Model file for the job. Use its own axes, mm. A direction names the side the tool comes from. Round coordinates to 2 decimals unless told otherwise and drop trailing zeros. Order: outer loops, then holes, each group sorted by start corner. A loop starts at its lowest first (then second) coordinate and runs counter-clockwise, first axis right, second up. Notation, with made-up numbers: (25, -7.75) - (36, -7.75) arc R17 ccw to (36, 12.25) - close; hole circle Ø9 at (-28.75, 44.25). An arc over 180 degrees is marked (long way). Put each result on its own line as item: value. Start each with the question number.
Item 1: Saw through at C-C on x = 100. List the corners of the cut face in (y, z).
Item 2: Which spindle directions (+Z, -Z, +X, -X, +Y, -Y) get a long thin tool onto all of the face, cutting with end or side? Do faces 1 (the face through (80, 14, 0)), 2 (the face through (80, 12.5, -82)). Say none if no direction does.
Item 3: Probe probe 1 along Z at (x, y) = (130, 8.5); probe 2 along X at (y, z) = (8.75, -9); probe 3 along Z at (x, y) = (19.5, 17.5). List the from-to ranges inside material, lowest first.
Item 4: Pin check, flat tip, straight feed: pin 1 Ø12 at (x, z) = (85.5, -82.5) entering from +Y. Stop position of the tip, or through.
Item 5: Saw through at A-A on z = -43. List the corners of the cut face in (x, y).
Item 6: Saw through at B-B on y = 19.75. List the corners of the cut face in (x, z), plus the area to 4 significant figures.
Item 7: Mould opens along X. For faces 3 (the face through (0, 14, -82)), 4 (the face through (80, 10, -11.5)), 5 (the face through (82, 1, -2)) say: pulls with the +X half, pulls with the -X half, needs draft (parallel to the pull), parting line crosses it, or undercut.
```python
from build123d import *

# Parameters (mm, degrees)
SKETCH1_W           = 162
SKETCH1_H           = 162
SKETCH1_W_2         = 140
SKETCH1_H_2         = 140
BOSS_EXTRUDE1_DEPTH = 7.5
SKETCH2_W           = 139
SKETCH2_H           = 139
BOSS_EXTRUDE2_DEPTH = 5
FILLET1_R           = 5
BOSS_EXTRUDE3_START = 15
BOSS_EXTRUDE3_DEPTH = 15


with BuildPart() as part:
    # Sketch1 → Boss-Extrude1 (new body)
    # profile 1 of 2: a face of its own
    with BuildSketch(Plane(origin=(0, 0, 0), x_dir=(1, 0, 0), z_dir=(0, 1, 0))):
        with Locations((81, 81)):
            Rectangle(SKETCH1_W, SKETCH1_H)
        with Locations((81, 81)):
            Rectangle(SKETCH1_W_2, SKETCH1_H_2, mode=Mode.SUBTRACT)
    # profile 2 of 2: a face of its own
    with BuildSketch(Plane(origin=(0, 0, 0), x_dir=(1, 0, 0), z_dir=(0, 1, 0))):
        with Locations((81, 81)):
            Rectangle(SKETCH1_W_2, SKETCH1_H_2)
    extrude(amount=BOSS_EXTRUDE1_DEPTH)

    # Sketch2 → Boss-Extrude2 (add)
    with BuildSketch(Plane(origin=(0, 7.5, 0), x_dir=(1, 0, 0), z_dir=(0, 1, 0))):
        with Locations((81, 81)):
            Rectangle(SKETCH2_W, SKETCH2_H)
    extrude(amount=BOSS_EXTRUDE2_DEPTH)

    # Fillet1
    fillet1_edges = [part.edges().sort_by_distance(p)[0] for p in [
        (11.5, 10, -150.5),
        (11.5, 10, -11.5),
        (150.5, 10, -11.5),
        (150.5, 10, -150.5),
        (0, 0, -81),
        (81, 0, -162),
        (162, 0, -81),
        (81, 0, 0),
        (0, 3.75, 0),
        (0, 3.75, -162),
        (162, 3.75, -162),
        (162, 3.75, 0),
    ]]
    fillet(fillet1_edges, radius=FILLET1_R)

    # Sketch3 → Boss-Extrude3 (add)
    with BuildSketch(Plane(origin=(0, 7.5, 0), x_dir=(1, 0, 0), z_dir=(0, 1, 0)).offset(BOSS_EXTRUDE3_START)):
        with BuildLine():
            ThreePointArc((5, 162), (1.464466094, 160.535533906), (0, 157))
            Line((0, 157), (0, 5))
            ThreePointArc((0, 5), (1.464466094, 1.464466094), (5, 0))
            Line((5, 0), (157, 0))
            ThreePointArc((157, 0), (160.535533906, 1.464466094), (162, 5))
            Line((162, 5), (162, 157))
            ThreePointArc((162, 157), (160.535533906, 160.535533906), (157, 162))
            Line((157, 162), (5, 162))
        make_face()
        with BuildLine():
            ThreePointArc((9.5, 157.5), (5.964466094, 156.035533906), (4.5, 152.5))
            Line((4.5, 152.5), (4.5, 9.5))
            ThreePointArc((4.5, 9.5), (5.964466094, 5.964466094), (9.5, 4.5))
            Line((9.5, 4.5), (152.5, 4.5))
            ThreePointArc((152.5, 4.5), (156.035533906, 5.964466094), (157.5, 9.5))
            Line((157.5, 9.5), (157.5, 152.5))
            ThreePointArc((157.5, 152.5), (156.035533906, 156.035533906), (152.5, 157.5))
            Line((152.5, 157.5), (9.5, 157.5))
        make_face(mode=Mode.SUBTRACT)
    extrude(amount=-BOSS_EXTRUDE3_DEPTH)


solid = part.part
```
Results found:
1. outline: (0, -157) arc R5 ccw to (5, -162) - (22.5, -162) - (22.5, -157.5) - (7.5, -157.5) - (7.5, -150.5) - (12.5, -150.5) - (12.5, -11.5) - (7.5, -11.5) - (7.5, -4.5) - (22.5, -4.5) - (22.5, 0) - (5, 0) arc R5 ccw to (0, -5) - close
2. face 1: +Z, +X, -X, +Y, -Y
2. face 2: +Y
3. probe 1: z = -162 to -157.5, -150.5 to -11.5, -4.5 to 0
3. probe 2: x = 0 to 4.53, 157.47 to 162
3. probe 3: z = -162 to -157.5, -4.5 to 0
4. pin 1: stops at y = 12.5
5. outline: (0, 5) arc R5 ccw to (5, 0) - (157, 0) arc R5 ccw to (162, 5) - (162, 22.5) - (157.5, 22.5) - (157.5, 7.5) - (150.5, 7.5) - (150.5, 12.5) - (11.5, 12.5) - (11.5, 7.5) - (4.5, 7.5) - (4.5, 22.5) - (0, 22.5) - close
6. outline: (0, -157) arc R5 ccw to (5, -162) - (157, -162) arc R5 ccw to (162, -157) - (162, -5) arc R5 ccw to (157, 0) - (5, 0) arc R5 ccw to (0, -5) - close; hole (4.5, -152.5) arc R5 ccw to (9.5, -157.5) - (152.5, -157.5) arc R5 ccw to (157.5, -152.5) - (157.5, -9.5) arc R5 ccw to (152.5, -4.5) - (9.5, -4.5) arc R5 ccw to (4.5, -9.5) - close
6. area: 2,835 mm²
7. face 3: pulls with the -X half
7. face 4: undercut
7. face 5: needs draft
